Verification items for the finished model (mm, model axes). A direction names the side the tool comes from. Coordinates: 2 decimals unless noted, no trailing zeros. Order: outer loops, then holes, each group sorted by start corner. A loop starts at its lowest first (then second) coordinate and runs counter-clockwise, first axis right, second up. Notation, with made-up numbers: (62.25, -33.75) -> (109.25, -33.75) arc R7 ccw to (109.25, -22.75) -> close; hole circle Ø7 at (5, -27). An arc over 180 degrees is marked (long way). Answer as CSV lines item,"result".
Autodesk Inventor part; units mm, degrees
ref_plane "body_screw_XY" through (0, -8, 3) normal (0, 0, 1) x (1, 0, 0)
ref_plane "body_screw_YZ" through (0, -8, 3) normal (1, 0, 0) x (0, 1, 0)
ref_plane "body_screw_ZX" through (0, -8, 3) normal (0, 1, 0) x (0, 0, 1)
sketch "Sketch_1" plane through (0, 0, 0) normal (0, 0, 1) x (1, 0, 0)
  line L0 (3, 0) -> (-3, 0)
  line L1 (-3, 12) -> (-3, 5.5)
  line L2 (-3, 5.5) -> (-2.5, 5)
  line L3 (-2.5, 5) -> (2.5, 5)
  line L4 (2.5, 5) -> (3, 5.5)
  line L5 (3, 5.5) -> (3, 12)
  line L6 (3, 12) -> (2.5, 12.5)
  line L7 (2.5, 12.5) -> (-2.5, 12.5)
  line L8 (-2.5, 12.5) -> (-3, 12)
revolve "Revolution1" add sketch "Sketch_1" angle 360 about axis through (3, 0, 0) along (1, 0, 0)
sketch "Sketch_2" plane through (0, 0, 0) normal (1, 0, 0) x (0, 1, 0)
  line L0 (-12.5, 0.75) -> (-12.5, -0.75)
  line L1 (-12.5, -0.75) -> (9, -0.75)
  line L2 (9, -0.75) -> (9, 0.75)
  line L3 (9, 0.75) -> (-12.5, 0.75)
extrude "Extrusion1" cut sketch "Sketch_2" along normal mid plane 6
sketch "Sketch_3" plane through (0, 0, 0) normal (1, 0, 0) x (0, 1, 0)
  line L0 (-8, 12.5) -> (-8, 0)
  line L1 (-8, 0) -> (-9.45, 0)
  line L2 (-9.45, 0) -> (-9.45, 3)
  line L3 (-9.45, 3) -> (-10.45, 3)
  line L4 (-10.45, 3) -> (-10.45, 12.5)
  line L5 (-10.45, 12.5) -> (-8, 12.5)
  line L6 (-8, 12.5) -> (-8, 0)
revolve "Revolution2" cut sketch "Sketch_3" angle 360 about axis through (0, -8, 12.5) along (0, 0, 1)
sketch "Sketch_4" plane through (0, 0, 0) normal (1, 0, 0) x (0, 1, 0)
  line L0 (-8, -12.75) -> (-8, -0.75)
  line L1 (-8, -0.75) -> (-6.75, -0.75)
  line L2 (-6.75, -0.75) -> (-6.9935, -0.9935)
  line L3 (-6.9935, -0.9935) -> (-6.9935, -12.75)
  line L4 (-6.9935, -12.75) -> (-8, -12.75)
  line L5 (-8, -12.75) -> (-8, -0.75)
revolve "Revolution3" cut sketch "Sketch_4" angle 360 about axis through (0, -8, -12.75) along (0, 0, -1)
thread "Thread1"
sketch "Sketch_7" plane through (0, 0, -9) normal (0, 0, 1) x (1, 0, 0)
  line L0 (3, 0) -> (-3, 0)
  line L1 (-3, 0) -> (-3, 1.5)
  line L2 (-3, 1.5) -> (-2.7295, 1.2295)
  line L3 (-2.7295, 1.2295) -> (2.7295, 1.2295)
  line L4 (2.7295, 1.2295) -> (3, 1.5)
  line L5 (3, 1.5) -> (3, 0)
  line L6 (3, 0) -> (-3, 0)
revolve "Revolution4" cut sketch "Sketch_7" angle 360 about axis through (3, 0, -9) along (1, 0, 0)
thread "Thread2"
sketch "Sketch_8" plane through (0, 0, 9) normal (0, 0, 1) x (1, 0, 0)
  line L0 (3, 0) -> (-3, 0)
  line L1 (-3, 0) -> (-3, 1.5)
  line L2 (-3, 1.5) -> (-2.7295, 1.2295)
  line L3 (-2.7295, 1.2295) -> (2.7295, 1.2295)
  line L4 (2.7295, 1.2295) -> (3, 1.5)
  line L5 (3, 1.5) -> (3, 0)
  line L6 (3, 0) -> (-3, 0)
revolve "Revolution5" cut sketch "Sketch_8" angle 360 about axis through (3, 0, 9) along (1, 0, 0)
thread "Thread3"
ref_plane "body_screw_XY" through (0, -8, 3) normal (0, 0, 1) x (1, 0, 0)
ref_plane "body_screw_YZ" through (0, -8, 3) normal (1, 0, 0) x (0, 1, 0)
ref_plane "body_screw_ZX" through (0, -8, 3) normal (0, 1, 0) x (0, 0, 1)
properties part number "SCSWJ10-6_b"
Item 1: Section check A-A, the plane y = 0. Count the separate pieces of the cut face and the enclosed holes in it, plus the area to 3 significant figures.
Answer list:
separate pieces,"4"
enclosed holes,"0"
area,"59.2 mm2"
Item 2: Section check B-B, the plane x = 0. Record the boundary of the cut face in (y, z).
Answer list:
outline,"(-12.48, -0.75) arc R12.5 ccw to (-9.01, -8.67) -> (-9.01, -0.99) -> (-9.25, -0.75) -> close; (-12.48, 0.75) -> (-9.45, 0.75) -> (-9.45, 3) -> (-10.45, 3) -> (-10.45, 6.86) arc R12.5 ccw to start; (-6.99, -10.36) arc R12.5 ccw (long way) to (-5.55, 11.2) -> (-5.55, 3) -> (-6.55, 3) -> (-6.55, 0.75) -> (-4.94, 0.75) arc R5 cw to (4.94, 0.75) -> (9, 0.75) -> (9, -0.75) -> (4.94, -0.75) arc R5 cw to (-4.94, -0.75) -> (-6.75, -0.75) -> (-6.99, -0.99) -> close; hole circle Ø2.46 at (0, -9); hole circle Ø2.46 at (0, 9)"
Item 3: Section check C-C, the plane x = 1.75. Record the boundary of the cut face in (y, z), plus the area to 3 significant figures.
Answer list:
outline,"(-12.48, -0.75) arc R12.5 ccw (long way) to (-6.29, 10.8) -> (-6.29, 3) -> (-9.71, 3) -> (-9.71, 7.87) arc R12.5 ccw to (-12.48, 0.75) -> (-4.94, 0.75) arc R5 cw to (4.94, 0.75) -> (9, 0.75) -> (9, -0.75) -> (4.94, -0.75) arc R5 cw to (-4.94, -0.75) -> close; hole circle Ø2.46 at (0, -9); hole circle Ø2.46 at (0, 9)"
area,"363 mm2"
Item 4: Tool access check on faces 5 (the cylindrical face through (0.3, -7.04, -5.74)), 6 (the cylindrical face through (0, 0, 5)), 7 (the cylindrical face through (0.108, -5.552, 6.247)), 8 (the flat face through (0, 7, 0.75)), 9 (the conical face through (2.64, 0.1, 5.14)). Record the directions out of +Z, -Z, +X, -X, +Y, -Y that give a thin tool (end or side, any length) a straight path to the whole face; none if there is none.
Answer list:
face 5,"+Z, -Z"
face 6,"+X, -X"
face 7,"+Z"
face 8,"+X, -X, -Y"
face 9,"+X"
Item 5: Thickness scan on line 1 (Z direction, x = 0.2, y = 0); line 2 (X direction, y = -8, z = 1.75); line 3 (Y direction, x = -0.5, z = 1). Record the ranges inside material, lowest first.
Answer list:
line 1,"-12.5 to -10.23, -7.77 to -5, 5 to 7.77, 10.23 to 12.5"
line 2,"-3 to -1.45, 1.45 to 3"
line 3,"-12.46 to -9.36, -6.64 to -4.9, 4.9 to 12.46"
Item 6: Release check for a two-part mould opening along Y. For faces 1 (the conical face through (-2.64, 0.1, -5.14)), 2 (the conical face through (-2.86, 12.13, -0.52)), 3 (the conical face through (-2.64, -0.1, 5.14)), 4 (the flat face through (-3, 5.2, -2.5)) record: +Y half, -Y half, draft (parallel to the pull), parting line (faces both ways), or undercut.
Answer list:
face 1,"undercut"
face 2,"parting line"
face 3,"undercut"
face 4,"draft"
Item 7: Depth check by flat-ended pin: pin 1 Ø2 at (y, z) = (0, 9) entering from +X; pin 2 Ø1.5 at (x, z) = (0, 9.5) entering from -Y; pin 3 Ø2 at (x, z) = (-0.5, 2) entering from +Y; pin 4 Ø2 at (x, z) = (0, 10) entering from -Y. Enter the tip coordinate at first touch or a pass-through.
Answer list:
pin 1,"through"
pin 2,"y = -5.67"
pin 3,"y = 12.46"
pin 4,"y = -5.76"
